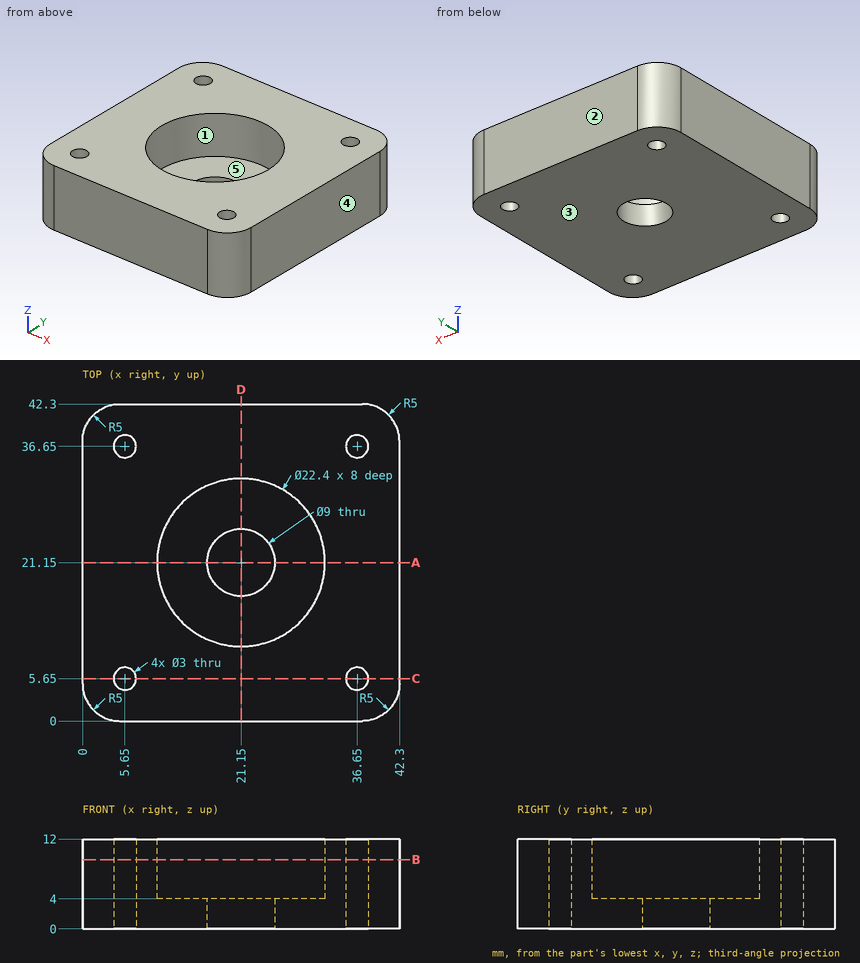
Drawing for the job (mm, zero at the part's lowest x, y, z). A direction names the side the tool comes from. Give positions to 0.01 mm unless a question says otherwise; leave off trailing zeros. Write each loop counter-clockwise with the first axis right and the second up, starting at its lowest first coordinate (ties: lowest second). Pieces come first, ordered by that corner, then holes. Notation, with made-up numbers: M 15.25,62 L 46.25,62 A13 ccw 46.25,71 Z; hole C 64,64.25 d2. An arc over 180 degrees is marked long. Use CSV: the item, a comma, the result in double quotes.
Item 1: Slice it at A-A on y = 21.15. Write the cut outline in (x, z).
Taken from the geometry:
outline,"M 0,0 L 16.65,0 L 16.65,4 L 9.95,4 L 9.95,12 L 0,12 Z; M 25.65,0 L 42.3,0 L 42.3,12 L 32.35,12 L 32.35,4 L 25.65,4 Z"
Item 2: Which spindle directions (+Z, -Z, +X, -X, +Y, -Y) get a long thin tool onto all of the face, cutting with end or side? Do the marked faces 4 and 5. Say none if no direction does.
Taken from the geometry:
face 4,"+Z, -Z, +X, +Y, -Y"
face 5,"+Z"
Item 3: Pin check, flat tips, straight feed: P1, Ø18, axis at x = 21.15, y = 21.15, coming from the +Z side; P2, Ø2.5, axis at x = 36.65, y = 36.65, coming from the +Z side. Stop position of each tip, or through.
Taken from the geometry:
P1,"stops at z = 4"
P2,"passes through"
Item 4: Slice it at B-B on z = 9.25. Write the cut outline in (x, y).
Taken from the geometry:
outline,"M 0,5 A5 ccw 5,0 L 37.3,0 A5 ccw 42.3,5 L 42.3,37.3 A5 ccw 37.3,42.3 L 5,42.3 A5 ccw 0,37.3 Z; hole C 5.65,5.65 d3; hole C 5.65,36.65 d3; hole C 21.15,21.15 d22.4; hole C 36.65,5.65 d3; hole C 36.65,36.65 d3"
Item 5: Drill centre lines: probe 1 along Y at (x, z) = (5.65, 4.75); probe 2 along X at (y, z) = (11, 9.75); probe 3 along Y at (x, z) = (17, 6.25). Where is each one in solid material? Low to high.
Taken from the geometry:
probe 1,"y = 0 to 4.15, 7.15 to 35.15, 38.15 to 42.3"
probe 2,"x = 0 to 16.42, 25.88 to 42.3"
probe 3,"y = 0 to 10.75, 31.55 to 42.3"
Item 6: Pull direction Y, two halves, no side cores. Call the marked faces 1, 2 and 3: +Y half, -Y half, draft (parallel to the pull), parting line (faces both ways), or undercut.
Taken from the geometry:
face 1,"undercut"
face 2,"+Y half"
face 3,"draft"
Item 7: Slice it at C-C on y = 5.65. Write the cut outline in (x, z).
Taken from the geometry:
outline,"M 0,0 L 4.15,0 L 4.15,12 L 0,12 Z; M 7.15,0 L 35.15,0 L 35.15,12 L 7.15,12 Z; M 38.15,0 L 42.3,0 L 42.3,12 L 38.15,12 Z"
